```python
from build123d import *

# Parameters (mm, degrees)
SALIENTE_EXTRUIR1_DEPTH = 13
REDONDEO1_R             = 13
VACIADO1_START          = -17
VACIADO1_3_DEPTH        = 17
VACIADO1_4_DEPTH        = 17


with BuildPart() as part:
    # Croquis1 → Saliente-Extruir1 (new body)
    with BuildSketch(Plane(origin=(0, 0, 0), x_dir=(0, 0, -1), z_dir=(1, 0, 0))):
        with BuildLine():
            Line((0, -35), (-17, -35))
            ThreePointArc((-17, -35), (-29.727922061, -29.727922061), (-35, -17))
            Line((-35, -17), (-35, 0))
            ThreePointArc((-35, 0), (24.748737342, 24.748737342), (0, -35))
        make_face()
    extrude(amount=SALIENTE_EXTRUIR1_DEPTH)

    # Redondeo1
    redondeo1_edges = [part.edges().sort_by_distance(p)[0] for p in [
        (0, -35, 8.5),
        (0, -29.727922061, 29.727922061),
        (0, -8.5, 35),
        (0, 24.748737342, -24.748737342),
    ]]
    fillet(redondeo1_edges, radius=REDONDEO1_R - 0.0001)  # a hair under: the kernel refuses the full size

    # Vaciado1: read off the stored shape, not the designer's step
    # Vaciado1 outline → Vaciado1 (revolve, cut)
    with BuildSketch(Plane(origin=(0, -17, 17), x_dir=(0, 1, 0), z_dir=(0, 0, -1))):
        with BuildLine():
            Line((0, 13), (0, 2))
            Line((0, 2), (5, 2))
            ThreePointArc((5, 2), (12.778174593, 5.221825407), (16, 13))
            Line((16, 13), (0, 13))
        make_face()
    revolve(axis=Axis((0, -17, 17), (1, 0, 0)), mode=Mode.SUBTRACT)

    # Vaciado1 2 outline → Vaciado1 2 (revolve, cut)
    with BuildSketch(Plane.YX):
        with BuildLine():
            Line((33, 13), (0, 13))
            Line((0, 13), (0, 2))
            Line((0, 2), (22, 2))
            ThreePointArc((22, 2), (29.778174593, 5.221825407), (33, 13))
        make_face()
    revolve(axis=Axis((0, 0, 0), (1, 0, 0)), mode=Mode.SUBTRACT)

    # Vaciado1 3 outline → Vaciado1 3 (cut)
    with BuildSketch(Plane(origin=(0, 0, 0), x_dir=(1, 0, 0), z_dir=(0, 1, 0)).offset(VACIADO1_START)):
        with BuildLine():
            ThreePointArc((2, -22), (5.221825407, -29.778174593), (13, -33))
            Line((13, -33), (13, -9))
            Line((13, -9), (2, -9))
            Line((2, -9), (2, -22))
        make_face()
    extrude(amount=VACIADO1_3_DEPTH, mode=Mode.SUBTRACT)

    # Vaciado1 4 outline → Vaciado1 4 (cut)
    with BuildSketch(Plane.XY):
        with BuildLine():
            ThreePointArc((2, -22), (5.221825407, -29.778174593), (13, -33))
            Line((13, -33), (13, 1))
            Line((13, 1), (2, 1))
            Line((2, 1), (2, -22))
        make_face()
    extrude(amount=VACIADO1_4_DEPTH, mode=Mode.SUBTRACT)


solid = part.part
```
Geometry check sheet. Reference: the model listing, model coordinates, mm. A direction names the side the tool comes from. Give positions to 0.01 mm unless a question says otherwise; leave off trailing zeros. Use a Markdown table: item, result.
Q1. Draft check along Y on faces 3 (the face through (3.909, -31.293, 8.619)), 4 (the face through (13, -34, 2)), 5 (the face through (5.137, -8.619, 29.692)). Enter one of: pulls with the +Y half, pulls with the -Y half, needs draft (parallel to the pull), parting line crosses it, or undercut.
Computed:
| item | result |
|---|---|
| face 3 | pulls with the -Y half |
| face 4 | needs draft |
| face 5 | undercut |
Q2. Thickness scan on L1, parallel to X at y = -8.5, z = 3; L2, parallel to Z at x = 8.25, y = 18.5; L3, parallel to Z at x = 8, y = 25.5. Record the ranges inside material, lowest first. Write a range as [from, to].
Computed:
| item | result |
|---|---|
| L1 | x = [0, 2] |
| L2 | z = [-28.65, -26.01], [26.01, 28.65] |
| L3 | z = [-22.49, -19], [19, 22.49] |
Q3. Set-up check for faces 1 (the face through (3.909, -8.381, 31.293)), 2 (the face through (5.137, -29.692, 8.381)): record each of +Z, -Z, +X, -X, +Y, -Y from which the full face is reachable in a straight line by a thin tool's end or side.
Computed:
| item | result |
|---|---|
| face 1 | +Z, -X, +Y, -Y |
| face 2 | +X |
Q4. Go/stop test with flat-tipped pins: P1, Ø1.5, axis at x = 9, y = -5, coming from the +Z side; P2, Ø3, axis at y = 11.5, z = 9.5, coming from the +X side; P3, Ø2, axis at x = 4.5, y = -25, coming from the -Z side. Record where each tip stops, or that it passes through.
Computed:
| item | result |
|---|---|
| P1 | stops at z = 34.59 |
| P2 | stops at x = 2 |
| P3 | stops at z = -21.45 |
